Input: part model. Units: mm. Frame: model coordinates. A direction names the side the tool comes from. Round coordinates to 2 decimals unless told otherwise and drop trailing zeros. Write each loop counter-clockwise with the first axis right and the second up, starting at its lowest first coordinate (ties: lowest second). Pieces come first, ordered by that corner, then holes. Notation, with made-up numbers: (29.5, 39.5) -> (52.5, 39.5) arc R23 ccw to (52.5, 59.5) -> close; hole circle Ø6 at (63.25, -11.75). An arc over 180 degrees is marked (long way). Write item = value, one per line.
```python
from build123d import *

# Parameters (mm, degrees)
SKETCH1_W          = 158.75
SKETCH1_H          = 35.56
EXTRUDE1_DEPTH     = 3.175
SKETCH3_W          = 19.05
SKETCH3_H          = 3.175
CUT_EXTRUDE1_DEPTH = 4.175


with BuildPart() as part:
    # Sketch1 → Extrude1 (new body)
    with BuildSketch(Plane(origin=(0, 0, 0), x_dir=(1, 0, 0), z_dir=(0, 1, 0))):
        Rectangle(SKETCH1_W, SKETCH1_H)
    extrude(amount=EXTRUDE1_DEPTH)

    # Sketch3 → Cut-Extrude1 (cut, through all)
    with BuildSketch(Plane(origin=(0, 3.175, 0), x_dir=(1, 0, 0), z_dir=(0, 1, 0))):
        Polygon((47.625, -14.605), (66.675, -14.605), (79.375, -14.605), (79.375, -17.78), (66.675, -17.78), (47.625, -17.78), align=None)
        with Locations((-69.85, 16.1925)):
            Rectangle(SKETCH3_W, SKETCH3_H)
        Polygon((66.675, 17.78), (79.375, 17.78), (79.375, 14.605), (66.675, 14.605), (47.625, 14.605), (47.625, 17.78), align=None)
        with Locations((25.4, -16.1925)):
            Rectangle(SKETCH3_W, SKETCH3_H)
        with Locations((-6.35, -16.1925)):
            Rectangle(SKETCH3_W, SKETCH3_H)
        with Locations((-38.1, -16.1925)):
            Rectangle(SKETCH3_W, SKETCH3_H)
        with Locations((-69.85, -16.1925)):
            Rectangle(SKETCH3_W, SKETCH3_H)
        with Locations((-38.1, 16.1925)):
            Rectangle(SKETCH3_W, SKETCH3_H)
        with Locations((-6.35, 16.1925)):
            Rectangle(SKETCH3_W, SKETCH3_H)
        with Locations((25.4, 16.1925)):
            Rectangle(SKETCH3_W, SKETCH3_H)
    extrude(amount=-CUT_EXTRUDE1_DEPTH, mode=Mode.SUBTRACT)


solid = part.part
```
1) First-contact query: P1, Ø1.6, axis at y = 1, z = 16, coming from the -X side (3 decimals); P2, Ø1.6, axis at y = 2, z = 16.5, coming from the +X side (3 decimals); P3, Ø1, axis at x = 28.5, y = 2.5, coming from the +Z side (3 decimals). Flat tips, straight axial feed; report the tip coordinate or a pass-through.
Solutions:
P1 = -60.325
P2 = 47.625
P3 = 14.605
2) Cut plane A-A (x = -40). Return the cut outline in (y, z) (3 decimals).
Solutions:
outline = (0, -14.605) -> (3.175, -14.605) -> (3.175, 14.605) -> (0, 14.605) -> close
3) Draft query along X for faces 1 (the face through (25, 2, -14.605)), 2 (the face through (79.375, 2, 0)), 3 (the face through (41, 2, 17.78)), 4 (the face through (34.925, 2, 16)). Return one class per face: +X half, -X half, draft (parallel to the pull), parting line (faces both ways), or undercut.
Solutions:
face_1 = undercut
face_2 = +X half
face_3 = draft
face_4 = undercut
4) Access query for faces 5 (the face through (64, 2, 14.605)), 6 (the face through (15.875, 2, -16)), 7 (the face through (-60.325, 2, 16)), 8 (the face through (47.625, 2, -16)). Directions: +Z, -Z, +X, -X, +Y, -Y. A direction counts if a zero-diameter tool reaches every point of the face in a straight line with its end or side. Return the directions, or none.
Solutions:
face_5 = +Z, +X, +Y, -Y
face_6 = -Z, +Y, -Y
face_7 = +Z, -X, +Y, -Y
face_8 = -Z, +X, +Y, -Y
5) Line query: L1, parallel to Z at x = -12.5, y = 1.6 (3 decimals). Output: solid intervals per line, ascending. Write a range as from..to.
Solutions:
L1 = -14.605..14.605
